Source: CAD feature listing. Evaluate the final solid. Frame: model axes, mm. A direction names the side the tool comes from. Coordinates: 2 decimals unless noted, no trailing zeros. Loops run counter-clockwise (first coordinate to the right, second up) from the corner with the lowest first, then second, coordinate; pieces in that order, holes last.
Item 1: Line query: probe 1 along Y at (x, z) = (22, -7); probe 2 along Y at (x, z) = (10, 19); probe 3 along Z at (x, y) = (13, -6). Output: solid intervals per line, ascending.
Item 2: Section query D-D, the plane z = 21. Return the cut outline in (x, y), then the cut area to 3 significant figures.
Item 3: Section query A-A, the plane x = 0. Return the cut outline in (y, z).
Item 4: Section query B-B, the plane z = 0. Return the cut outline in (x, y), then the cut area to 3 significant figures.
Item 5: Section query C-C, the plane y = -26. Return the cut outline in (x, z), then the cut area to 3 significant figures.
Item 6: Reachability of faces 1 (the flat face through (0, 0, 0)), 2 (the flat face through (-22.34, -60, 3.82)), 3 (the flat face through (-11, -50, 17)) from +Z, -Z, +X, -X, +Y, -Y: full face, straight path, thin tool, end or side. Return the list, or none.
Item 7: Pin query (flat end, axial travel): pin 1 Ø8 at (x, y) = (-17.5, -13.5) entering from +Z; pin 2 Ø10 at (y, z) = (-46.5, -15) entering from +X; pin 3 Ø1.5 at (y, z) = (-14.5, -17) entering from +X. Return the tip coordinate at first contact, or that it passes through.
```python
from build123d import *

# Parameters (mm, degrees)
F0_R     = 20
F1_DEPTH = 50
F2_R     = 25
F3_DEPTH = 10
F4_R     = 22.5
F5_DEPTH = 10
F6_R     = 1


with BuildPart() as f1:
    # F0 (on Front) → F1 (new body)
    with BuildSketch(Plane.XZ):
        Circle(F0_R)
    extrude(amount=F1_DEPTH)

    # F2 (on face) → F3 (join)
    with BuildSketch(Plane.XZ.offset(50)):
        Circle(F2_R)
    extrude(amount=F3_DEPTH)

    # F4 (on face) → F5 (join)
    with BuildSketch(Plane.XZ.offset(60)):
        Circle(F4_R)
    extrude(amount=F5_DEPTH)

    # F6
    f6_edges = [f1.edges().sort_by_distance(p)[0] for p in [
        (-20, 0, 0),
    ]]
    fillet(f6_edges, radius=F6_R)


solid = f1.part
```
Verdict:
1. probe 1: y = -60 to -50
1. probe 2: y = -70 to -50
1. probe 3: z = -15.2 to 15.2
2. outline: (-13.56, -60) - (-8.08, -60) - (-8.08, -70) - (8.08, -70) - (8.08, -60) - (13.56, -60) - (13.56, -50) - (-13.56, -50) - close
2. area: 433 mm2
3. outline: (-70, -22.5) - (-60, -22.5) - (-60, -25) - (-50, -25) - (-50, -20) - (-1, -20) arc R1 ccw to (0, -19) - (0, 19) arc R1 ccw to (-1, 20) - (-50, 20) - (-50, 25) - (-60, 25) - (-60, 22.5) - (-70, 22.5) - close
4. outline: (-25, -60) - (-22.5, -60) - (-22.5, -70) - (22.5, -70) - (22.5, -60) - (25, -60) - (25, -50) - (20, -50) - (20, -1) arc R1 ccw to (19, 0) - (-19, 0) arc R1 ccw to (-20, -1) - (-20, -50) - (-25, -50) - close
4. area: 2,950 mm2
5. outline: circle Ø40 at (0, 0)
5. area: 1,260 mm2
6. face 1: +Z, -Z, +X, -X, +Y
6. face 2: -Y
6. face 3: +Y
7. pin 1: stops at z = 14.76
7. pin 2: stops at x = 22.23
7. pin 3: stops at x = 11.66
